For this review, take the finished solid that the model builds, in its own axes (mm). Face numbers are marked on the shaded views. A direction names the side the tool comes from. Give positions to 0.01 mm unless a question says otherwise; leave off trailing zeros. Loops run counter-clockwise (first coordinate to the right, second up) from the corner with the lowest first, then second, coordinate; pieces in that order, holes last.
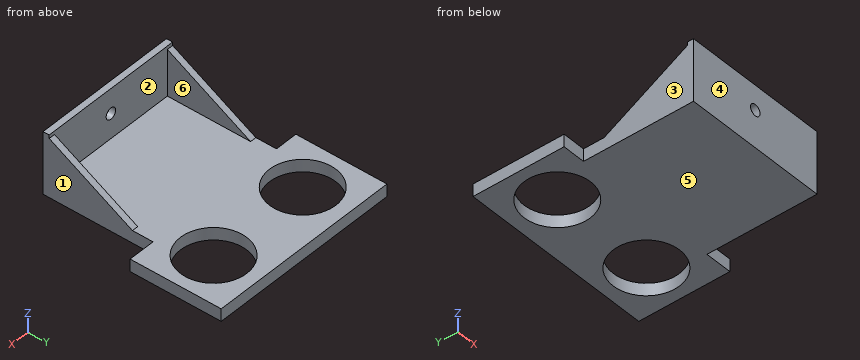
```python
from build123d import *

# Parameters (mm, degrees)
BOSS_EXTRUDE3_DEPTH = 1.5
BOSS_EXTRUDE4_DEPTH = 1.5
SKETCH2_W           = 35
SKETCH2_H           = 12
SKETCH2_R           = 1.35
BOSS_EXTRUDE7_DEPTH = 1.5
SKETCH3_R           = 8
BOSS_EXTRUDE8_DEPTH = 3


with BuildPart() as part:
    # Sketch5 → Boss-Extrude3 (new body)
    with BuildSketch(Plane(origin=(-17.5, 0, 0), x_dir=(0, 1, 0), z_dir=(-1, 0, 0))):
        Polygon((21.59, 6), (0, -6), (0, 6), align=None)
    extrude(amount=-BOSS_EXTRUDE3_DEPTH)



with BuildPart() as body_2:
    # Sketch4 → Boss-Extrude4 (new body)
    with BuildSketch(Plane(origin=(17.5, 0, 0), x_dir=(0, 0, -1), z_dir=(1, 0, 0))):
        Polygon((6, 21.592468158), (-6, 0), (6, 0), align=None)
    extrude(amount=-BOSS_EXTRUDE4_DEPTH)


with BuildPart() as part_1:
    add(part.part)

    add(body_2.part)  # Boss-Extrude7 merges body 2
    # Sketch2 → Boss-Extrude7 (add)
    with BuildSketch(Plane(origin=(0, 0, 0), x_dir=(1, 0, 0), z_dir=(0, 1, 0))):
        Rectangle(SKETCH2_W, SKETCH2_H)
        with Locations(Location((0, 0, 0), (0, 0, 270))):
            Circle(SKETCH2_R, mode=Mode.SUBTRACT)
    extrude(amount=BOSS_EXTRUDE7_DEPTH)

    # Sketch3 → Boss-Extrude8 (add)
    with BuildSketch(Plane(origin=(0, 0, -6), x_dir=(-1, 0, 0), z_dir=(0, 0, -1))):
        Polygon((17.5, 0), (-17.5, 0), (-17.5, 26.57366529), (-23.990187259, 26.57366529), (-23.990187259, 48.57366529), (23.009812741, 48.57366529), (23.009812741, 26.57366529), (17.5, 26.57366529), align=None)
        with Locations((-13.240187259, 37.57366529)):
            Circle(SKETCH3_R, mode=Mode.SUBTRACT)
        with Locations(Location((12.259812741, 37.374598913, 0), (0, 0, 180))):
            Circle(SKETCH3_R, mode=Mode.SUBTRACT)
    extrude(amount=BOSS_EXTRUDE8_DEPTH)


solid = part_1.part
```
Q1. For probe 1 along X at (y, z) = (43, -7.5); probe 2 along Y at (x, z) = (3, -2.75); probe 3 along Z at (x, y) = (-6, 25.5), list the stretches that pass through material, from the lowest coordinate up.
Answers:
probe 1: x = -23.01 to -17.95, -6.57 to 7.36, 19.12 to 23.99
probe 2: y = 0 to 1.5
probe 3: z = -9 to -6
Q2. Consider section C-C on y = 14. Give the boundary of the cut face in (x, z), plus the area to 3 significant figures.
Answers:
outline: (-17.5, -9) - (17.5, -9) - (17.5, -1.78) - (16, -1.78) - (16, -6) - (-16, -6) - (-16, -1.78) - (-17.5, -1.78) - close
area: 118 mm2
Q3. For pin 1 Ø1 at (y, z) = (7.5, -6) entering from -X; pin 2 Ø9 at (y, z) = (13, -2) entering from +X; pin 3 Ø3 at (x, z) = (0, 0) entering from +Y, all flat-tipped, find the tip position at first contact; note any pin that passes through.
Answers:
pin 1: stops at x = -17.5
pin 2: stops at x = 17.5
pin 3: stops at y = 1.5
Q4. Consider section B-B on z = 0. Give the boundary of the cut face in (x, y) (3 decimals), plus the area to 3 significant figures.
Answers:
outline: (-17.5, 0) - (-1.35, 0) - (-1.35, 1.5) - (-16, 1.5) - (-16, 10.795) - (-17.5, 10.795) - close; (1.35, 0) - (17.5, 0) - (17.5, 10.796) - (16, 10.796) - (16, 1.5) - (1.35, 1.5) - close
area: 76.3 mm2
Q5. Consider section A-A on x = 0. Give the boundary of the cut face in (y, z).
Answers:
outline: (0, -9) - (48.57, -9) - (48.57, -6) - (1.5, -6) - (1.5, -1.35) - (0, -1.35) - close; (0, 1.35) - (1.5, 1.35) - (1.5, 6) - (0, 6) - close
Q6. Consider section D-D on z = -7.5. Give the boundary of the cut face in (x, y).
Answers:
outline: (-23.01, 26.57) - (-17.5, 26.57) - (-17.5, 0) - (17.5, 0) - (17.5, 26.57) - (23.99, 26.57) - (23.99, 48.57) - (-23.01, 48.57) - close; hole circle Ø16 at (-12.26, 37.37); hole circle Ø16 at (13.24, 37.57)
Q7. Machinability: for the marked faces 5 and 6, which of the approach directions +Z, -Z, +X, -X, +Y, -Y give a long, thin tool a straight path to every point of the face, cutting with its end or side? Answer none if there is none.
Answers:
face 5: -Z, +X, -X, +Y, -Y
face 6: +Z, +Y
Q8. Mouldability with a two-part tool opening along X and no side actions: class the marked faces 1, 2, 3 and 4 as +X half, -X half, draft (parallel to the pull), parting line (faces both ways), or undercut.
Answers:
face 1: +X half
face 2: undercut
face 3: -X half
face 4: draft
